from build123d import *

# Parameters (mm, degrees)
F0_R     = 25
F0_R_2   = 10
F1_DEPTH = 15
F2_R     = 5
F3_R     = 3
F4_R     = 5
F5_R     = 3
F6_R     = 1
F7_DEPTH = 12
F8_DEPTH = 1


with BuildPart() as f1:
    # F0 (on Front) → F1 (new body)
    with BuildSketch(Plane.XZ):
        Circle(F0_R)
        Circle(F0_R_2, mode=Mode.SUBTRACT)
    extrude(amount=F1_DEPTH)

    # F2
    f2_edges = [f1.edges().sort_by_distance(p)[0] for p in [
        (-25, -15, 0),
    ]]
    fillet(f2_edges, radius=F2_R)

    # F3
    f3_edges = [f1.edges().sort_by_distance(p)[0] for p in [
        (-10, -15, 0),
    ]]
    fillet(f3_edges, radius=F3_R)

    # F4
    f4_edges = [f1.edges().sort_by_distance(p)[0] for p in [
        (-25, 0, 0),
    ]]
    fillet(f4_edges, radius=F4_R)

    # F5
    f5_edges = [f1.edges().sort_by_distance(p)[0] for p in [
        (-10, 0, 0),
    ]]
    fillet(f5_edges, radius=F5_R)

    # F6 (on Front) → F7 (join)
    with BuildSketch(Plane.XZ):
        with BuildLine():
            Line((-0.5, 9.9874921777), (-0.5, 1.3737387097))
            Line((-0.5, 1.3737387097), (-6.0368140021, 7.9722566883))
            ThreePointArc((-6.0368140021, 7.9722566883), (-6.4278760969, 7.6604444312), (-6.8028584452, 7.3294690786))
            Line((-6.8028584452, 7.3294690786), (-1.2660444431, 0.7309511))
            Line((-1.2660444431, 0.7309511), (-9.7489356409, 2.2267136926))
            ThreePointArc((-9.7489356409, 2.2267136926), (-9.8480775301, 1.7364817767), (-9.9225838186, 1.2419059396))
            Line((-9.9225838186, 1.2419059396), (-1.4396926208, -0.253856653))
            Line((-1.4396926208, -0.253856653), (-8.899421946, -4.560733387))
            ThreePointArc((-8.899421946, -4.560733387), (-8.6602540378, -5), (-8.399421946, -5.4267587908))
            Line((-8.399421946, -5.4267587908), (-0.9396926208, -1.1198820568))
            Line((-0.9396926208, -1.1198820568), (-3.8857698165, -9.2141626279))
            ThreePointArc((-3.8857698165, -9.2141626279), (-3.4202014333, -9.3969262079), (-2.9460771957, -9.5561827712))
            Line((-2.9460771957, -9.5561827712), (0, -1.4619022001))
            Line((0, -1.4619022001), (2.9460771957, -9.5561827712))
            ThreePointArc((2.9460771957, -9.5561827712), (3.4202014333, -9.3969262079), (3.8857698165, -9.2141626279))
            Line((3.8857698165, -9.2141626279), (0.9396926208, -1.1198820568))
            Line((0.9396926208, -1.1198820568), (8.399421946, -5.4267587908))
            ThreePointArc((8.399421946, -5.4267587908), (8.6602540378, -5), (8.899421946, -4.560733387))
            Line((8.899421946, -4.560733387), (1.4396926208, -0.253856653))
            Line((1.4396926208, -0.253856653), (9.9225838186, 1.2419059396))
            ThreePointArc((9.9225838186, 1.2419059396), (9.8480775301, 1.7364817767), (9.7489356409, 2.2267136926))
            Line((9.7489356409, 2.2267136926), (1.2660444431, 0.7309511))
            Line((1.2660444431, 0.7309511), (6.8028584452, 7.3294690786))
            ThreePointArc((6.8028584452, 7.3294690786), (6.4278760969, 7.6604444312), (6.0368140021, 7.9722566883))
            Line((6.0368140021, 7.9722566883), (0.5, 1.3737387097))
            Line((0.5, 1.3737387097), (0.5, 9.9874921777))
            ThreePointArc((0.5, 9.9874921777), (0, 10), (-0.5, 9.9874921777))
        make_face()
        Circle(F6_R, mode=Mode.SUBTRACT)
    extrude(amount=F7_DEPTH)

    # F6 (on Front) → F8 (cut)
    with BuildSketch(Plane.XZ):
        with BuildLine():
            Line((-0.5, 9.9874921777), (-0.5, 1.3737387097))
            Line((-0.5, 1.3737387097), (-6.0368140021, 7.9722566883))
            ThreePointArc((-6.0368140021, 7.9722566883), (-6.4278760969, 7.6604444312), (-6.8028584452, 7.3294690786))
            Line((-6.8028584452, 7.3294690786), (-1.2660444431, 0.7309511))
            Line((-1.2660444431, 0.7309511), (-9.7489356409, 2.2267136926))
            ThreePointArc((-9.7489356409, 2.2267136926), (-9.8480775301, 1.7364817767), (-9.9225838186, 1.2419059396))
            Line((-9.9225838186, 1.2419059396), (-1.4396926208, -0.253856653))
            Line((-1.4396926208, -0.253856653), (-8.899421946, -4.560733387))
            ThreePointArc((-8.899421946, -4.560733387), (-8.6602540378, -5), (-8.399421946, -5.4267587908))
            Line((-8.399421946, -5.4267587908), (-0.9396926208, -1.1198820568))
            Line((-0.9396926208, -1.1198820568), (-3.8857698165, -9.2141626279))
            ThreePointArc((-3.8857698165, -9.2141626279), (-3.4202014333, -9.3969262079), (-2.9460771957, -9.5561827712))
            Line((-2.9460771957, -9.5561827712), (0, -1.4619022001))
            Line((0, -1.4619022001), (2.9460771957, -9.5561827712))
            ThreePointArc((2.9460771957, -9.5561827712), (3.4202014333, -9.3969262079), (3.8857698165, -9.2141626279))
            Line((3.8857698165, -9.2141626279), (0.9396926208, -1.1198820568))
            Line((0.9396926208, -1.1198820568), (8.399421946, -5.4267587908))
            ThreePointArc((8.399421946, -5.4267587908), (8.6602540378, -5), (8.899421946, -4.560733387))
            Line((8.899421946, -4.560733387), (1.4396926208, -0.253856653))
            Line((1.4396926208, -0.253856653), (9.9225838186, 1.2419059396))
            ThreePointArc((9.9225838186, 1.2419059396), (9.8480775301, 1.7364817767), (9.7489356409, 2.2267136926))
            Line((9.7489356409, 2.2267136926), (1.2660444431, 0.7309511))
            Line((1.2660444431, 0.7309511), (6.8028584452, 7.3294690786))
            ThreePointArc((6.8028584452, 7.3294690786), (6.4278760969, 7.6604444312), (6.0368140021, 7.9722566883))
            Line((6.0368140021, 7.9722566883), (0.5, 1.3737387097))
            Line((0.5, 1.3737387097), (0.5, 9.9874921777))
            ThreePointArc((0.5, 9.9874921777), (0, 10), (-0.5, 9.9874921777))
        make_face()
        Circle(F6_R, mode=Mode.SUBTRACT)
    extrude(amount=F8_DEPTH, mode=Mode.SUBTRACT)


solid = f1.part
Geometry check sheet. Reference: the model listing, model coordinates, mm. A direction names the side the tool comes from. Give positions to 0.01 mm unless a question says otherwise; leave off trailing zeros.
(1) Thickness scan on L1, parallel to Z at x = -5, y = -3.25; L2, parallel to Z at x = -5, y = -2.25; L3, parallel to X at y = -3, z = -5.5. Record the ranges inside material, lowest first.
From the geometry:
L1: z = -24.17 to -8.66, -3.46 to -2.31, 0.37 to 1.39, 5.18 to 6.74, 8.66 to 24.17
L2: z = -23.65 to -8.77, -3.46 to -2.31, 0.37 to 1.39, 5.18 to 6.74, 8.77 to 23.65
L3: x = -23.96 to -8.35, -2.53 to -1.47, 1.47 to 2.53, 8.35 to 23.96
(2) Release check for a two-part mould opening along Z. For faces 1 (the flat face through (-4.722, -6.423, -3.303)), 2 (the cylindrical face through (23.846, -7.465, 7.509)), 3 (the flat face through (4, 0, -13)) record: released by +Z, released by -Z, zero draft, split by the parting line, or undercut.
From the geometry:
face 1: undercut
face 2: split by the parting line
face 3: zero draft
(3) Set-up check for faces 4 (the flat face through (4, -15, -13)), 5 (the cylindrical face through (-8.639, -7.437, 5.036)): record each of +Z, -Z, +X, -X, +Y, -Y from which the full face is reachable in a straight line by a thin tool's end or side.
From the geometry:
face 4: +Z, -Z, +X, -X, -Y
face 5: +Y, -Y
(4) Depth check by flat-ended pin: pin 1 Ø5 at (y, z) = (-5.5, -5.5) entering from -X; pin 2 Ø3 at (x, y) = (9, -11.5) entering from +Z; pin 3 Ø2.5 at (x, z) = (0, 0) entering from -Y; pin 4 Ø21.5 at (x, z) = (4, 4.5) entering from +Y. Enter the tip coordinate at first touch or a pass-through.
From the geometry:
pin 1: stops at x = -24.82
pin 2: stops at z = 23.73
pin 3: stops at y = -12
pin 4: stops at y = 0
(5) Section check A-A on y = -9. Count the separate pieces of the cut face and the enclosed holes in it, then the cut area to 3 significant figures.
From the geometry:
separate pieces: 1
enclosed holes: 10
area: 1,730 mm2
